```python
from build123d import *

# Parameters (mm, degrees)
BOSS_EXTRUDE1_DEPTH                                 = 40
FILLET1_R                                           = 20
CUT_EXTRUDE2_REACH                                  = 150.682
SKETCH3_R                                           = 12
SKETCH4_R                                           = 10
CUT_EXTRUDE3_DEPTH                                  = 7
CIRPATTERN1_COUNT                                   = 12
F_10_0_10_DIAMETER_HOLE1_D                          = 10
SKETCH8_R                                           = 8.5
CUT_EXTRUDE4_DEPTH                                  = 23
CBORE_FOR_M6_HEX_SOCKET_HEAD_CAP_SCREW1_D           = 6.4
CBORE_FOR_M6_HEX_SOCKET_HEAD_CAP_SCREW1_CBORE_D     = 11
CBORE_FOR_M6_HEX_SOCKET_HEAD_CAP_SCREW1_CBORE_DEPTH = 6.4
F_8_0MM_DOWEL_HOLE1_D                               = 8
CHAMFER1_SIZE                                       = 1
CHAMFER2_SIZE                                       = 0.5
CHAMFER3_SIZE                                       = 1


with BuildPart() as part:
    # Sketch1 → Boss-Extrude1 (new body)
    with BuildSketch(Plane(origin=(0, 0, 0), x_dir=(1, 0, 0), z_dir=(0, 1, 0))):
        with BuildLine():
            Line((-90, 0), (-90, 39.504902432))
            ThreePointArc((-90, 39.504902432), (-85.182396525, 94.862332258), (-30.561841884, 84.652075111))
            ThreePointArc((-30.561841884, 84.652075111), (0, 90), (30.561841884, 84.652075111))
            ThreePointArc((30.561841884, 84.652075111), (85.182396525, 94.862332258), (90, 39.504902432))
            Line((90, 39.504902432), (90, 0))
            ThreePointArc((90, 0), (0, -90), (-90, 0))
        make_face()
    extrude(amount=-BOSS_EXTRUDE1_DEPTH)

    # Fillet1
    fillet1_edges = [part.edges().sort_by_distance(p)[0] for p in [
        (30.561841884, -20, -84.652075111),
        (90, -20, -39.504902432),
        (-90, -20, -39.504902432),
        (-30.561841884, -20, -84.652075111),
    ]]
    fillet(fillet1_edges, radius=FILLET1_R)

    # Sketch3 → Cut-Extrude2 (cut, up to next)
    with BuildSketch(Plane(origin=(0, 0, 0), x_dir=(1, 0, 0), z_dir=(0, 1, 0)), mode=Mode.PRIVATE) as cut_extrude2_sk1:
        with Locations(Location((-62.5, 65, 0), (0, 0, 270))):
            Circle(SKETCH3_R)
    cut_extrude2_tool1 = extrude(cut_extrude2_sk1.sketch, amount=-CUT_EXTRUDE2_REACH, mode=Mode.PRIVATE) & part.part
    # Sketch3 → Cut-Extrude2 (cut, up to next)
    with BuildSketch(Plane(origin=(0, 0, 0), x_dir=(1, 0, 0), z_dir=(0, 1, 0)), mode=Mode.PRIVATE) as cut_extrude2_sk2:
        with Locations(Location((62.5, 65, 0), (0, 0, 270))):
            Circle(SKETCH3_R)
    cut_extrude2_tool2 = extrude(cut_extrude2_sk2.sketch, amount=-CUT_EXTRUDE2_REACH, mode=Mode.PRIVATE) & part.part
    add(cut_extrude2_tool1.solids().sort_by_distance((-62.5, 0, -65))[0], mode=Mode.SUBTRACT)
    add(cut_extrude2_tool2.solids().sort_by_distance((62.5, 0, -65))[0], mode=Mode.SUBTRACT)

    # Sketch4 → Cut-Extrude3 (cut)
    with BuildSketch(Plane(origin=(0, 0, 0), x_dir=(1, 0, 0), z_dir=(0, 1, 0))):
        with Locations(Location((0, 45, 0), (0, 0, 270))):
            Circle(SKETCH4_R)
    cut_extrude3 = extrude(amount=-CUT_EXTRUDE3_DEPTH, mode=Mode.SUBTRACT)

    # CirPattern1: Cut-Extrude3 ×12 about axis
    cirpattern1_axis = Axis((0, 0, 0), (0, 1, 0))
    for i in range(1, CIRPATTERN1_COUNT):
        add(cut_extrude3.rotate(cirpattern1_axis, i * 360 / CIRPATTERN1_COUNT), mode=Mode.SUBTRACT)

    # Ø10.0 (10) Diameter Hole1 (through all)
    with Locations(Plane(origin=(0, 0, 0), x_dir=(1, 0, 0), z_dir=(0, 1, 0))):
        with Locations((0, 45), (45, 0), (0, -45), (-45, 0)):
            Hole(F_10_0_10_DIAMETER_HOLE1_D / 2)

    # Sketch8 → Cut-Extrude4 (cut)
    with BuildSketch(Plane.XZ.offset(40)):
        with Locations(Location((0, 45, 0), (0, 0, 270))):
            Circle(SKETCH8_R)
        with Locations(Location((45, 0, 0), (0, 0, 270))):
            Circle(SKETCH8_R)
        with Locations(Location((0, -45, 0), (0, 0, 270))):
            Circle(SKETCH8_R)
        with Locations(Location((-45, 0, 0), (0, 0, 270))):
            Circle(SKETCH8_R)
    extrude(amount=-CUT_EXTRUDE4_DEPTH, mode=Mode.SUBTRACT)

    # CBORE for M6 Hex Socket Head Cap Screw1 (through all)
    with Locations(Plane(origin=(0, -40, 0), x_dir=(-1, 0, 0), z_dir=(0, -1, 0))):
        with Locations((0, 22.5), (-19.485571585, -11.25), (19.485571585, -11.25)):
            CounterBoreHole(CBORE_FOR_M6_HEX_SOCKET_HEAD_CAP_SCREW1_D / 2, CBORE_FOR_M6_HEX_SOCKET_HEAD_CAP_SCREW1_CBORE_D / 2, CBORE_FOR_M6_HEX_SOCKET_HEAD_CAP_SCREW1_CBORE_DEPTH)

    # Ø8.0mm Dowel Hole1 (through all)
    with Locations(Plane(origin=(0, 0, 0), x_dir=(1, 0, 0), z_dir=(0, 1, 0))):
        with Locations((-22.5, 0), (22.5, 0)):
            Hole(F_8_0MM_DOWEL_HOLE1_D / 2)

    # Chamfer1
    chamfer1_edges = [part.edges().sort_by_distance(p)[0] for p in [
        (0, -40, 90),
        (87.062864481, 0, -93.335766948),
        (87.062864481, -40, -93.335766948),
        (90, -40, -16.298148254),
        (0, 0, -90),
        (0, -40, -90),
        (-87.062864481, 0, -93.335766948),
        (-87.062864481, -40, -93.335766948),
        (-90, 0, -16.298148254),
        (-90, -40, -16.298148254),
        (28.863873105, 0, -88.103017476),
        (28.863873105, -40, -88.103017476),
        (-28.863873105, 0, -88.103017476),
        (-28.863873105, -40, -88.103017476),
        (90.889338282, 0, -38.493974754),
        (90.889338282, -40, -38.493974754),
        (-90.889338282, 0, -38.493974754),
        (-90.889338282, -40, -38.493974754),
        (-62.5, 0, -77),
        (-62.5, -40, -77),
        (62.5, 0, -77),
        (62.5, -40, -77),
        (90, 0, -16.298148254),
        (0, 0, 90),
    ]]
    chamfer(chamfer1_edges, length=CHAMFER1_SIZE)

    # Chamfer2
    chamfer2_edges = [part.edges().sort_by_distance(p)[0] for p in [
        (0, -40, 53.5),
        (45, -40, 8.5),
        (0, -40, -36.5),
        (-45, -40, 8.5),
    ]]
    chamfer(chamfer2_edges, length=CHAMFER2_SIZE)

    # Chamfer3
    chamfer3_edges = [part.edges().sort_by_distance(p)[0] for p in [
        (0, 0, -55),
        (-47.631397208, 0, -27.5),
        (-55, 0, 0),
        (-27.5, 0, 47.631397208),
        (-47.631397208, 0, 27.5),
        (55, 0, 0),
        (47.631397208, 0, 27.5),
        (27.5, 0, 47.631397208),
        (0, 0, 55),
        (27.5, 0, -47.631397208),
        (47.631397208, 0, -27.5),
        (-27.5, 0, -47.631397208),
    ]]
    chamfer(chamfer3_edges, length=CHAMFER3_SIZE)


solid = part.part
```
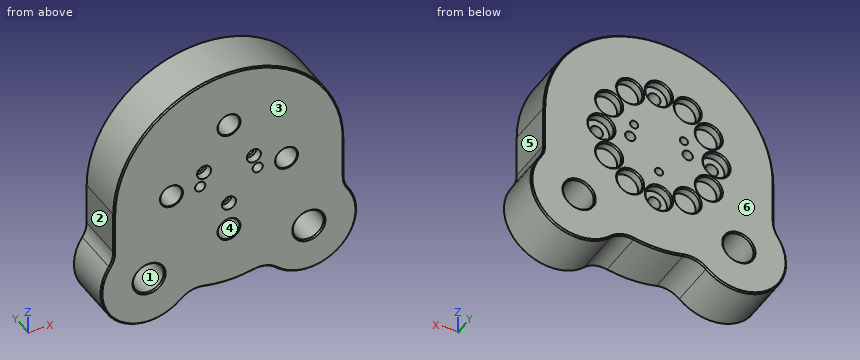
Could you check a few things on this model? Use its own coordinates, in mm. Face numbers are marked on the shaded views. A direction names the side the tool comes from. Coordinates: 2 decimals unless noted, no trailing zeros. Write each loop counter-clockwise with the first axis right and the second up, starting at its lowest first coordinate (ties: lowest second). Pieces come first, ordered by that corner, then holes. Notation, with made-up numbers: (-12, 58.25) - (11, 58.25) arc R26 cw to (11, 82.25) - close; hole circle Ø2 at (58.5, 32). An arc over 180 degrees is marked (long way). Use a Markdown table: item, result.
Q1. Which directions (+Z, -Z, +X, -X, +Y, -Y) give clear straight access to the entire face, cutting with the end or side of a thin tool? Please do the marked faces 4, 5 and 6.
Geometry check:
| item | result |
|---|---|
| face 4 | -Y |
| face 5 | +Z, +X, +Y, -Y |
| face 6 | +Z, -Z, +X, -X, +Y |
Q2. Imagine slicing it at B-B (y = -11). Count the separate pieces of the cut face and the enclosed holes in it, and give its area (3 significant figures).
Geometry check:
| item | result |
|---|---|
| separate pieces | 1 |
| enclosed holes | 11 |
| area | 29,100 mm2 |
Q3. Thinking about a two-plate mould opening in X: for the marked faces 1, 2 and 3, which applies, +X half, -X half, draft (parallel to the pull), parting line (faces both ways), or undercut?
Geometry check:
| item | result |
|---|---|
| face 1 | undercut |
| face 2 | -X half |
| face 3 | draft |
Q4. Please list where these lines run through material, in increasing order: L1, parallel to Z at x = 0, y = -12; L2, parallel to X at y = -36, z = -22.5; L3, parallel to X at y = -10, z = 11.
Geometry check:
| item | result |
|---|---|
| L1 | z = -90 to -50, -40 to -25.7, -19.3 to 40, 50 to 90 |
| L2 | x = -90 to -5.5, 5.5 to 90 |
| L3 | x = -89.33 to -22.68, -16.3 to 16.3, 22.68 to 89.33 |
Q5. I'm going to push flat-ended pins straight in: pin 1 Ø5 at (x, z) = (46.5, 0) entering from -Y; pin 2 Ø2 at (y, z) = (-9, 48) entering from +X; pin 3 Ø10 at (x, z) = (-23.5, -41) entering from +Y; pin 4 Ø8 at (y, z) = (-32.5, -24) entering from -X. Where does each tip first touch, or does it pass through?
Geometry check:
| item | result |
|---|---|
| pin 1 | passes through |
| pin 2 | stops at x = 76.75 |
| pin 3 | stops at y = -7 |
| pin 4 | stops at x = -90 |
Q6. Imagine slicing it at A-A (z = -65). List the corners of the cut face in (x, y) for me.
Geometry check:
| item | result |
|---|---|
| outline | (-100, -39) - (-99, -40) - (-75.5, -40) - (-74.5, -39) - (-74.5, -1) - (-75.5, 0) - (-99, 0) - (-100, -1) - close; (-50.5, -39) - (-49.5, -40) - (49.5, -40) - (50.5, -39) - (50.5, -1) - (49.5, 0) - (-49.5, 0) - (-50.5, -1) - close; (74.5, -39) - (75.5, -40) - (99, -40) - (100, -39) - (100, -1) - (99, 0) - (75.5, 0) - (74.5, -1) - close |
